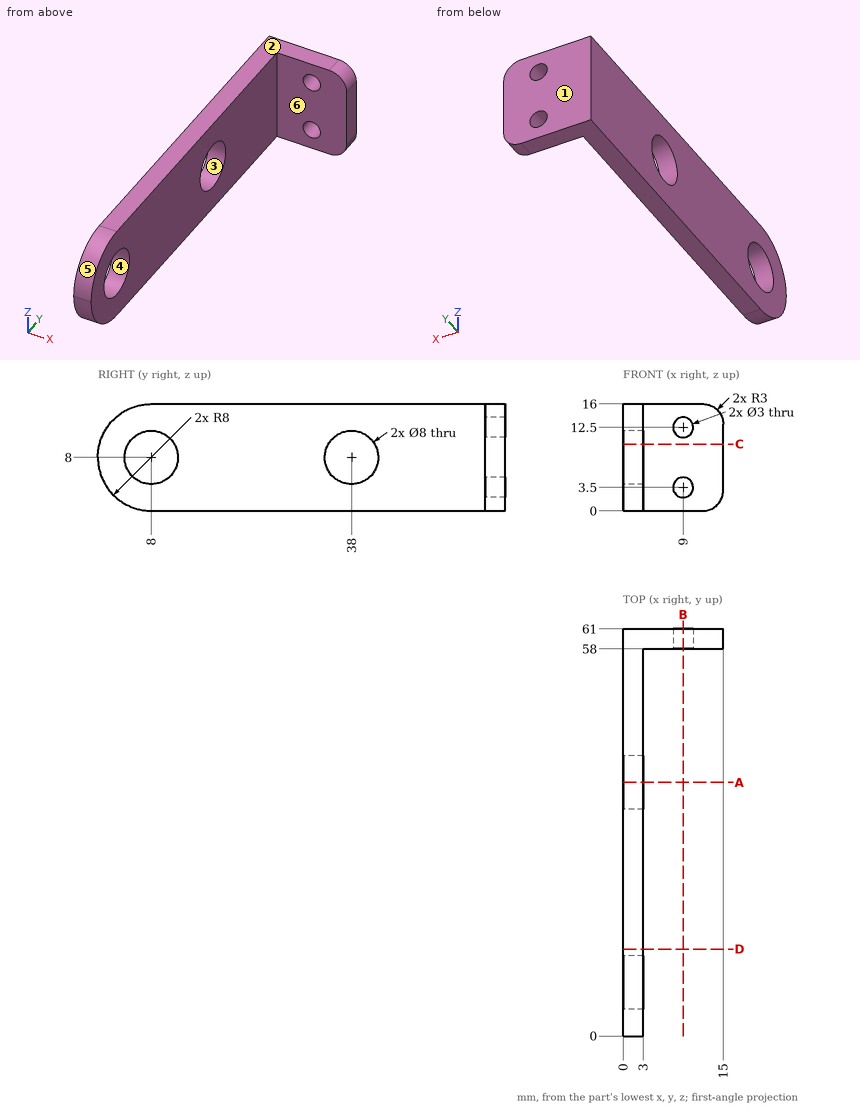
Study the drawing (mm; zero at the part's minimum x, y, z) and answer. A direction names the side the tool comes from. Give positions to 0.01 mm unless a question says otherwise; leave off trailing zeros. Write each loop counter-clockwise with the first axis right and the second up, starting at its lowest first coordinate (ties: lowest second). Pieces come first, ordered by that corner, then holes. Notation, with made-up numbers: (9, 50.5) -> (31, 50.5) arc R12 ccw to (31, 59.5) -> close; hole circle Ø6 at (43, 6.25). An arc over 180 degrees is marked (long way). Answer in a Markdown table with one row per item.
1) Section D-D on y = 13 is taken. Give the vertices of the cut face in (x, z).
Results list:
| item | result |
|---|---|
| outline | (0, 0) -> (3, 0) -> (3, 16) -> (0, 16) -> close |
2) Section B-B on x = 9 is taken. Give the vertices of the cut face in (y, z).
Results list:
| item | result |
|---|---|
| outline | (58, 0) -> (61, 0) -> (61, 2) -> (58, 2) -> close; (58, 5) -> (61, 5) -> (61, 11) -> (58, 11) -> close; (58, 14) -> (61, 14) -> (61, 16) -> (58, 16) -> close |
3) Determine the mould class of the marked faces 1, 2, 3 and 4 for opening direction Z: released by +Z, released by -Z, zero draft, split by the parting line, or undercut.
Results list:
| item | result |
|---|---|
| face 1 | zero draft |
| face 2 | released by +Z |
| face 3 | undercut |
| face 4 | undercut |
4) A tool of negligible diameter and unlimited length cuts with its end or side. For the marked faces 5 and 6, from which of +Z, -Z, +X, -X, +Y, -Y can it reach the whole face along a straight path? Write none if from no direction.
Results list:
| item | result |
|---|---|
| face 5 | +Z, +X, -X, -Y |
| face 6 | +Z, -Z, +X, -Y |
5) Straight lines are drawn through the part: line 1 (Z direction, x = 9, y = 59.7); line 2 (Y direction, x = 0.9, z = 8); line 3 (X direction, y = 60.25, z = 12.5). For each, find the intervals that lie inside material, in ascending order. Write a range as [from, to].
Results list:
| item | result |
|---|---|
| line 1 | [0, 2], [5, 11], [14, 16] |
| line 2 | [0, 4], [12, 34], [42, 61] |
| line 3 | [0, 7.5], [10.5, 15] |
6) Each of these flat-tipped pins is pushed along its axis until it touches: pin 1 Ø6 at (x, z) = (9, 10.5) entering from -Y; pin 2 Ø2 at (x, y) = (5, 49.5) entering from +Z; pin 3 Ø6 at (y, z) = (23.5, 6.5) entering from +X. Where does it stop, or does it pass through?
Results list:
| item | result |
|---|---|
| pin 1 | y = 58 |
| pin 2 | through |
| pin 3 | x = 3 |
7) Section C-C on z = 10 is taken. Give the vertices of the cut face in (x, y) (1 decimal).
Results list:
| item | result |
|---|---|
| outline | (0, 0.3) -> (3, 0.3) -> (3, 4.5) -> (0, 4.5) -> close; (0, 11.5) -> (3, 11.5) -> (3, 34.5) -> (0, 34.5) -> close; (0, 41.5) -> (3, 41.5) -> (3, 58) -> (15, 58) -> (15, 61) -> (0, 61) -> close |
8) Section A-A on y = 38 is taken. Give the vertices of the cut face in (x, z).
Results list:
| item | result |
|---|---|
| outline | (0, 0) -> (3, 0) -> (3, 4) -> (0, 4) -> close; (0, 12) -> (3, 12) -> (3, 16) -> (0, 16) -> close |
